from build123d import *

# Parameters (mm, degrees)
BOSS_EXTRUDE1_DEPTH = 80
SKETCH2_R           = 2.5
CUT_EXTRUDE1_DEPTH  = 21
CUT_EXTRUDE2_DEPTH  = 10


with BuildPart() as part:
    # Sketch1 → Boss-Extrude1 (new body)
    with BuildSketch(Plane.XY):
        Polygon((0, 0), (20, 0), (20, 3), (3, 3), (3, 60), (0, 60), align=None)
    extrude(amount=BOSS_EXTRUDE1_DEPTH)

    # Sketch2 → Cut-Extrude1 (cut, through all)
    with BuildSketch(Plane.ZY):
        with Locations((40, 30)):
            Circle(SKETCH2_R)
    extrude(amount=-CUT_EXTRUDE1_DEPTH, mode=Mode.SUBTRACT)

    # Sketch3 → Cut-Extrude2 (cut)
    with BuildSketch(Plane.ZY):
        with BuildLine():
            ThreePointArc((57.758584744, 56.445517931), (63.433655861, 54.048079801), (67.628756298, 49.536397843))
            ThreePointArc((67.628756298, 49.536397843), (66.763094992, 46.108478576), (63.335175725, 46.974139881))
            ThreePointArc((63.335175725, 46.974139881), (60.566344139, 49.951920199), (56.820708869, 51.534266681))
            ThreePointArc((56.820708869, 51.534266681), (54.834021181, 54.458830243), (57.758584744, 56.445517931))
        make_face()
    extrude(amount=-CUT_EXTRUDE2_DEPTH, mode=Mode.SUBTRACT)


solid = part.part
Could you check a few things on this model? Use its own coordinates, in mm. A direction names the side the tool comes from. Give positions to 0.01 mm unless a question says otherwise; leave off trailing zeros. Order: outer loops, then holes, each group sorted by start corner. A loop starts at its lowest first (then second) coordinate and runs counter-clockwise, first axis right, second up.
Item 1: If we section it at D-D, the plane x = 13.75: Write out the boundary of the cut face in (y, z), plus the area to 3 significant figures.
Item 2: If we section it at C-C, the plane z = 11.5: Write out the boundary of the cut face in (x, y), plus the area to 3 significant figures.
Item 3: If we section it at B-B, the plane z = 40: Write out the boundary of the cut face in (x, y), plus the area to 3 significant figures.
Item 4: If we section it at A-A, the plane y = 30: Write out the boundary of the cut face in (x, z).
Item 5: I need wall thicknesses on line 1 (Y direction, x = 1.05, z = 40); line 2 (Y direction, x = 17, z = 24). Which ranges of each line are inside material? Lowest first, please.
Item 6: If we mould it in two halves opening along Z, with no side actions, what happens to faces 4 (the face through (2.5, 25.7, 80)), 5 (the face through (1.479, 54.405, 54.824)), 6 (the face through (12, 3, 39)), 7 (the face through (2.5, 25.7, 0))? For each: pulls with the +Z half, pulls with the -Z half, needs draft (parallel to the pull), parting line crosses it, or undercut.
Item 7: I'm going to push flat-ended pins straight in: pin 1 (5 mm diameter, centred on y = 29, z = 14, fed in from +X); pin 2 (3 mm diameter, centred on y = 30, z = 40, fed in from +X). Where does each tip first touch, or does it pass through?
Item 8: For faces 1 (the face through (2, 60, 39)), 2 (the face through (3, 25, 39)), 3 (the face through (1.48, 49.92, 60.61)), which set-ups out of +Z, -Z, +X, -X, +Y, -Y let a thin tool reach every point of the face, with its end or its side?
Values:
1. outline: (0, 0) - (3, 0) - (3, 80) - (0, 80) - close
1. area: 240 mm2
2. outline: (0, 0) - (20, 0) - (20, 3) - (3, 3) - (3, 60) - (0, 60) - close
2. area: 231 mm2
3. outline: (0, 0) - (20, 0) - (20, 3) - (3, 3) - (3, 27.5) - (0, 27.5) - close; (0, 32.5) - (3, 32.5) - (3, 60) - (0, 60) - close
3. area: 216 mm2
4. outline: (0, 0) - (3, 0) - (3, 37.5) - (0, 37.5) - close; (0, 42.5) - (3, 42.5) - (3, 80) - (0, 80) - close
5. line 1: y = 0 to 27.5, 32.5 to 60
5. line 2: y = 0 to 3
6. face 4: pulls with the +Z half
6. face 5: undercut
6. face 6: needs draft
6. face 7: pulls with the -Z half
7. pin 1: stops at x = 3
7. pin 2: passes through
8. face 1: +Z, -Z, +X, -X, +Y
8. face 2: +Z, -Z, +X, +Y
8. face 3: +X, -X
